Job drawing, mm, ordinate dimensions from the low corner. One solid piece. A direction names the side the tool comes from. Round coordinates to 2 decimals unless told otherwise and drop trailing zeros. Write each loop counter-clockwise with the first axis right and the second up, starting at its lowest first coordinate (ties: lowest second). Pieces come first, ordered by that corner, then holes. Notation, with made-up numbers: M 46,-3.75 L 93,-3.75 A16 ccw 93,25.25 Z; hole C -17.5,0.5 d2. An arc over 180 degrees is marked long. One line per item, written item: value. Start each with the question number.
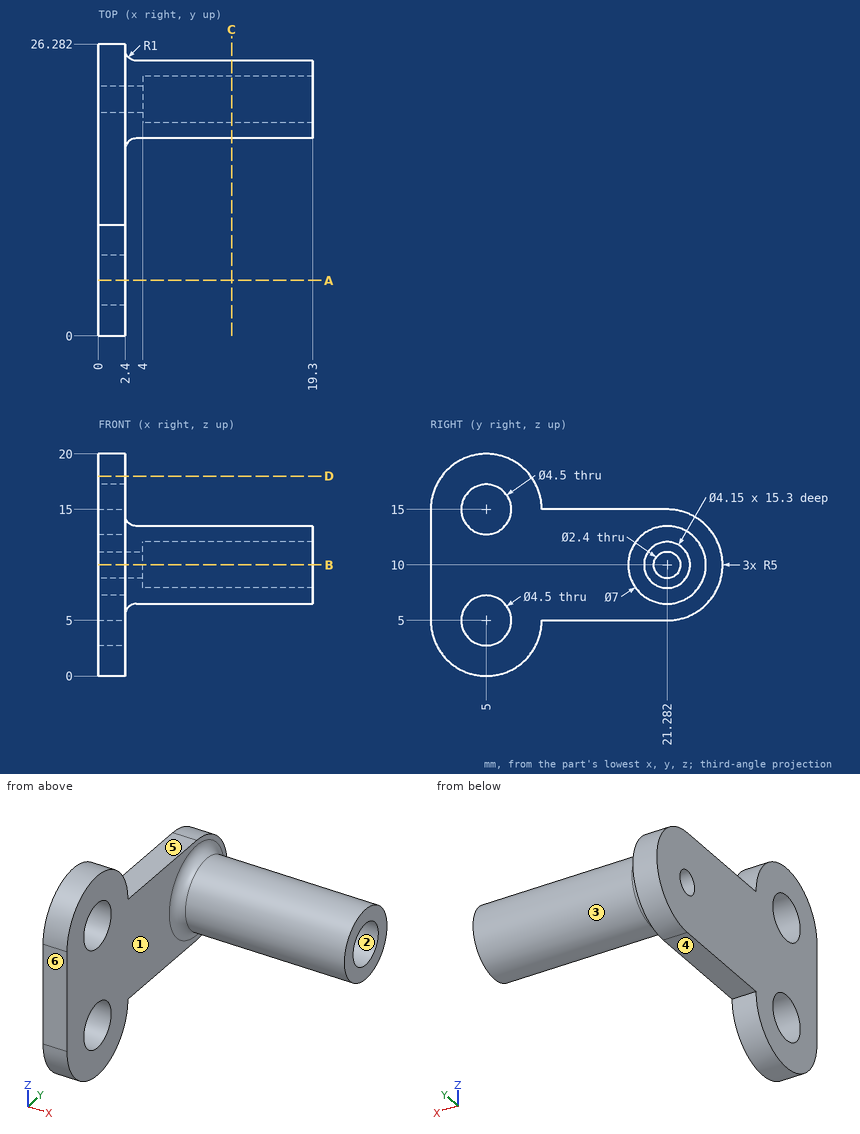
Item 1: Drill centre lines: line 1 (Y direction, x = 8.5, z = 10); line 2 (X direction, y = 1.75, z = 3.75); line 3 (Z direction, x = 1, y = 11.75). Where is each one in solid material? Low to high.
Item 2: Which spindle directions (+Z, -Z, +X, -X, +Y, -Y) get a long thin tool onto all of the face, cutting with end or side? Do the marked faces 4, 5 and 6. Say none if no direction does.
Item 3: Cut at D-D, the plane z = 18. Write the cut outline in (x, y).
Item 4: Cut at A-A, the plane y = 5. Write the cut outline in (x, z).
Item 5: Cut at C-C, the plane x = 12. Write the cut outline in (y, z) (3 decimals).
Item 6: Two-plate mould, pull along Y, no slides. Class the marked faces 1, 2 and 3: pulls with the +Y half, pulls with the -Y half, needs draft (parallel to the pull), parting line crosses it, or undercut.
Item 7: Drop flat-ended pins along their axis: pin 1 (4 mm diameter, centred on x = 8.5, z = 14, fed in from +Y); pin 2 (0.7 mm diameter, centred on x = 2, y = 15.5, fed in from -Z); pin 3 (3 mm diameter, centred on y = 21.28, z = 10, fed in from +X); pin 4 (1.5 mm diameter, centred on x = 8, y = 17, fed in from -Z). Give the stop position or say it passes through.
Item 8: Cut at B-B, the plane z = 10. Write the cut outline in (x, y).
Computed values:
1. line 1: y = 17.78 to 19.21, 23.36 to 24.78
1. line 2: x = 0 to 2.4
1. line 3: z = 5 to 15
2. face 4: -Z, +X, -X, +Y
2. face 5: +Z, +X, -X, +Y
2. face 6: +Z, -Z, +X, -X, -Y
3. outline: M 0,1 L 2.4,1 L 2.4,9 L 0,9 Z
4. outline: M 0,0 L 2.4,0 L 2.4,2.75 L 0,2.75 Z; M 0,7.25 L 2.4,7.25 L 2.4,12.75 L 0,12.75 Z; M 0,17.25 L 2.4,17.25 L 2.4,20 L 0,20 Z
5. outline: C 21.282,10 d7; hole C 21.282,10 d4.15
6. face 1: needs draft
6. face 2: undercut
6. face 3: parting line crosses it
7. pin 1: stops at y = 24.15
7. pin 2: stops at z = 5
7. pin 3: stops at x = 4
7. pin 4: passes through
8. outline: M 0,0 L 2.4,0 L 2.4,16.78 A1 cw 3.4,17.78 L 19.3,17.78 L 19.3,19.21 L 4,19.21 L 4,20.08 L 0,20.08 Z; M 0,22.48 L 4,22.48 L 4,23.36 L 19.3,23.36 L 19.3,24.78 L 3.4,24.78 A1 cw 2.4,25.78 L 2.4,26.28 L 0,26.28 Z
